from build123d import *

# Parameters (mm, degrees)
F0_W     = 5.842
F0_H     = 12.7
F0_R     = 3.175
F2_DEPTH = 3.175
F2_TAPER = -3


# Not quite as in the source:
# - a feature names something its author has since deleted; it is built from what else it names


with BuildPart() as f1:
    # F0 (on Front) → F1 (revolve)
    with BuildSketch(Plane.XZ):
        with Locations((2.921, 6.35)):
            Rectangle(F0_W, F0_H)
        Polygon((5.842, 12.7), (5.842, 0), (66.294, 0), (66.294, 12.7), (56.134, 12.7), (56.134, 10.16), (10.16, 10.16), (10.16, 12.7), align=None)
    revolve(axis=Axis((33.147, 0, 0), (-1, 0, 0)))

    # F0 (on Front) → F2 (join, symmetric)
    with BuildSketch(Plane.XZ):
        with BuildLine():
            Line((-0.9398, 0), (0, 0))
            Line((0, 0), (0, 12.7))
            Line((0, 12.7), (5.842, 12.7))
            Line((5.842, 12.7), (5.842, 15.24))
            Line((5.842, 15.24), (-0.508, 15.24))
            Line((-0.508, 15.24), (-10.8806298187, 3.8475430269))
            ThreePointArc((-10.8806298187, 3.8475430269), (-4.5919612295, 5.3297205562), (-0.9398, 0))
        make_face()
        with BuildLine():
            ThreePointArc((-8.1826630726, -5.5069827884), (-3.1957909266, -4.5493385486), (-0.9398, 0))
            ThreePointArc((-0.9398, 0), (-4.5919612295, 5.3297205562), (-10.8806298187, 3.8475430269))
            ThreePointArc((-10.8806298187, 3.8475430269), (-12.1459778134, -1.5837270034), (-8.1826630726, -5.5069827884))
        make_face()
        with Locations((-6.6548, 0)):
            Circle(F0_R, mode=Mode.SUBTRACT)
        with BuildLine():
            Line((5.842, 0), (0, 0))
            Line((0, 0), (-0.9398, 0))
            ThreePointArc((-0.9398, 0), (-3.1957909266, -4.5493385486), (-8.1826630726, -5.5069827884))
            Line((-8.1826630726, -5.5069827884), (5.842, -9.398))
            Line((5.842, -9.398), (5.842, 0))
        make_face()
    extrude(amount=F2_DEPTH, both=True, taper=F2_TAPER)


solid = f1.part
Could you check a few things on this model? Use its own coordinates, in mm. A direction names the side the tool comes from. Coordinates: 2 decimals unless noted, no trailing zeros. Write each loop counter-clockwise with the first axis right and the second up, starting at its lowest first coordinate (ties: lowest second). Pieces come first, ordered by that corner, then holes. Notation, with made-up numbers: (85.5, -35.75) - (95.5, -35.75) arc R6 cw to (95.5, -26.75) - close; hole circle Ø11 at (26, -7.75). An arc over 180 degrees is marked (long way). Write item = value, one per line.
1) Will these pins go through, and if not, where does the flat tip stop? pin 1 Ø1.5 at (y, z) = (0, 4) entering from -X; pin 2 Ø5 at (x, y) = (17.5, 9.5) entering from +Z; pin 3 Ø10 at (x, z) = (40.5, 11.5) entering from +Y.
Result set:
pin_1 = -11.36
pin_2 = 7.36
pin_3 = 7.81
2) Please list where these lines run through material, in increasing order: line 1 (X direction, y = -11, z = -3.5); line 2 (Y direction, x = -5, z = 4) (3 decimals); line 3 (X direction, y = -8.25, z = -2.75). Write a range as [from, to].
Result set:
line_1 = [0, 10.16], [56.13, 66.29]
line_2 = [-3.175, 3.175]
line_3 = [0, 66.29]
3) Suppose I cut it at A-A on y = -8.75. Please give me the cut outline in (x, z).
Result set:
outline = (0, -9.2) - (10.16, -9.2) - (10.16, -5.16) - (56.13, -5.16) - (56.13, -9.2) - (66.29, -9.2) - (66.29, 9.2) - (56.13, 9.2) - (56.13, 5.16) - (10.16, 5.16) - (10.16, 9.2) - (0, 9.2) - close
4) For faces 4 (the flat face through (66.294, 0, 0)), 5 (the conical face through (-3.707, -1.61, -0.928)), which set-ups out of +Z, -Z, +X, -X, +Y, -Y let a thin tool reach every point of the face, with its end or its side?
Result set:
face_4 = +Z, -Z, +X, +Y, -Y
face_5 = none
5) We'd pull the mould along X, two halves only. Please class faces 1 (the flat face through (-4, 3.175, 3)), 2 (the flat face through (0, -5, 0)), 3 (the flat face through (10.16, 9, 6)): +X half, -X half, draft (parallel to the pull), parting line (faces both ways), or undercut.
Result set:
face_1 = draft
face_2 = -X half
face_3 = undercut
6) Suppose I cut it at B-B on x = 24.5. Please give me the cut outline in (y, z).
Result set:
outline = circle Ø20.32 at (0, 0)
